Autodesk Inventor part; units mm, degrees
ref_plane "YZ Plane" through (0, 0, 0) normal (1, 0, 0) x (0, 1, 0)
ref_plane "XZ Plane" through (0, 0, 0) normal (0, 1, 0) x (-1, 0, 0)
ref_plane "XY Plane" through (0, 0, 0) normal (0, 0, 1) x (1, 0, 0)
sketch "Sketch1" plane through (0, 0, 0) normal (0, 0, 1) x (1, 0, 0)
  circle A0 centre (-47.5, -10) radius 3
  circle A1 centre (-5, 30) radius 2
  line L0 (-47.5, -10) -> (-2.5, -10)
  line L1 (7.5, 0) -> (-12.5, 0)
  line L2 (-12.5, 0) -> (-12.5, -20)
  line L3 (-12.5, -20) -> (7.5, -20)
  line L4 (7.5, -20) -> (7.5, 0)
  line L5 (7.5, 0) -> (-12.5, -20) construction
  line L6 (-12.5, 0) -> (7.5, -20) construction
  point P0 (0, 0)
  dimension "d0" = 45
  dimension "d1" = 20
  dimension "d2" = 20
extrude "Extrusion1" add sketch "Sketch1" along normal blind 6 contours L4 L3 L2 L1
ref_plane "Work Plane1" through (0, 0, -20) normal (0, 0, -1) x (-1, 0, 0)
sketch "Sketch2" plane through (0, 0, -20) normal (0, 0, -1) x (-1, 0, 0)
  line L0 (-7.5, -20) -> (-7.5, 0)
  line L1 (-7.5, 0) -> (12.5, 0)
  line L2 (12.5, 0) -> (12.5, -20)
  line L3 (12.5, -20) -> (-7.5, -20)
  point P0 (0, 0)
  dimension "d0" = 45
  dimension "d1" = 20
  dimension "d2" = 20
extrude "Extrusion2" add sketch "Sketch2" along normal blind 6
ref_plane "Work Plane2" through (-8, 25, 15) normal (0, 0, 1) x (0, 1, 0)
sketch "Sketch3" plane through (-8, 25, 15) normal (0, 0, 1) x (0, 1, 0)
  circle A0 centre (5, -3) radius 2
  arc A1 (8, -10) -> (10, -8) centre (8, -8) ccw
  line L0 (10, -8) -> (10, -3)
  line L1 (10, -3) -> (10, 5)
  line L2 (0, 5) -> (10, 5)
  line L3 (0, 5) -> (0, -3)
  line L4 (0, -3) -> (0, -8)
  arc A2 (0, -8) -> (2, -10) centre (2, -8) ccw
  line L5 (8, -10) -> (2, -10)
  circle A3 centre (5, -3) radius 2
  line L6 (0, 4) -> (10, 4)
  line L7 (10, 4) -> (10, -10)
  line L8 (10, -10) -> (0, -10)
  line L9 (0, -10) -> (0, 4)
  line L10 (0, 4) -> (10, -10) construction
  line L11 (10, 4) -> (0, -10) construction
  point P0 (-25, -8)
  point P1 (0, -8)
  point P2 (2, -10)
  point P3 (10, -8)
  dimension "d7" = 10
  dimension "d8" = 14
extrude "Extrusion3" add sketch "Sketch3" along normal blind 6
sketch "Sketch4" plane through (-13, 25, 15) normal (0, -1, 0) x (1, 0, 0)
  line L0 (0, 0) -> (15, 0)
  line L1 (15, 0) -> (15, 6)
  line L2 (0, 6) -> (15, 6)
  line L3 (0, 0) -> (0, 6)
  point P0 (13, -15)
sketch "Sketch5" plane through (-12.5, 0, 0) normal (0, 1, 0) x (1, 0, 0)
  line L0 (20, 0) -> (0, 0)
  line L1 (0, 0) -> (0, -6)
  line L2 (20, -6) -> (0, -6)
  line L3 (20, 0) -> (20, -6)
  point P0 (12.5, 0)
loft "Loft1" add section 1 edges at (-2.5, 0, 0) (-12.5, 0, 3) (-2.5, 0, 6) (7.5, 0, 3) section 2 edges at (-5.5, 25, 15) (2, 25, 18) (-5.5, 25, 21) (-13, 25, 18)
ref_plane "Work Plane3" through (0, 0, -10) normal (0, 0, 1) x (1, 0, 0)
mirror "Mirror1" about plane through (0, 0, -10) normal (0, 0, 1) of "Extrusion3", "Loft1"
sketch "Sketch7" plane through (-12.5, -20, 0) normal (0, -1, 0) x (1, 0, 0)
  line L0 (0, 0) -> (20, 0)
  line L1 (20, 0) -> (20, 6)
  line L2 (0, 6) -> (20, 6)
  line L3 (0, 0) -> (0, 6)
  line L4 (20, -20) -> (0, -20)
  line L5 (0, -20) -> (0, -26)
  line L6 (20, -26) -> (0, -26)
  line L7 (20, -20) -> (20, -26)
  line L8 (20, -20) -> (20, -26)
  line L9 (0, 6) -> (20, 6)
  line L10 (20, 6) -> (20, -26)
  line L11 (20, -26) -> (0, -26)
  line L12 (0, -26) -> (0, 6)
  point P0 (12.5, 0)
extrude "Extrusion5" add sketch "Sketch7" along normal blind 5
sketch "Sketch8" plane through (0, 0, 6) normal (0, 0, 1) x (1, 0, 0)
  line L0 (-12.5, -20) -> (7.5, -20)
  line L1 (-2.5, -20) -> (-2.5, -10)
  circle A0 centre (-2.5, -10) radius 3
  point P0 (0, 0)
  dimension "d23" = 10
  dimension "d24" = 6
extrude "Extrusion6" cut sketch "Sketch8" against normal blind 40
fillet "Fillet1" radius 2 2 edges at (2, 35, 18) (2, 35, -38)
fillet "Fillet2" radius 4 2 edges at (-2.5, -25, 6) (-2.5, -25, -26)
sketch "Sketch9" plane through (-12.5, -25, 0) normal (0, -1, 0) x (1, 0, 0)
  line L0 (20, -22) -> (0, -22)
  line L1 (20, -22) -> (20, 2)
  line L2 (0, 2) -> (20, 2)
  line L3 (0, 2) -> (0, -22)
  line L4 (0, 2) -> (0, -22)
  line L5 (0, -22) -> (20, 2)
  line L6 (0, 2) -> (20, 2)
  line L7 (0, 2) -> (20, -22)
  circle A0 centre (10, -10) radius 3
  point P0 (12.5, 0)
  dimension "d29" = 6
extrude "Extrusion7" cut sketch "Sketch9" against normal blind 40 contours A0 L5 L7 | L7 L5 A0 | A0 L7 L5 | L5 L7 A0
properties part number "2020_fixer2"
Could you check a few things on this model? Use its own coordinates, in mm. A direction names the side the tool comes from. Round coordinates to 2 decimals unless told otherwise and drop trailing zeros. Order: outer loops, then holes, each group sorted by start corner. A loop starts at its lowest first (then second) coordinate and runs counter-clockwise, first axis right, second up. Notation, with made-up numbers: M 6.5,26 L 64.5,26 A12 ccw 64.5,38 Z; hole C 60.5,74 d10. An arc over 180 degrees is marked long. One line per question, with ' | ' between items. Start each with the question number.
(1) Please list where these lines run through material, in increasing order: line 1 along Z through (x, y) = (-6.75, -17.5); line 2 along X through (y, z) = (-10, 1.6); line 3 along X through (y, z) = (30, -39.15).
(2) For P1, Ø6.5, axis at x = -5, y = 30, coming from the -Z side; P2, Ø8, axis at x = -2.5, y = -10, coming from the -Z side; P3, Ø5, axis at y = 29, z = -38, coming from the +X side; P4, Ø10, axis at x = 2, y = -14, coming from the +Z side, each with a flat end and sliding along its axis, tell me the tip position at first contact or that it passes through.
(3) Suppose I cut it at A-A on y = 30. List the corners of the cut face in (x, z) for me, then the cut area to 3 significant figures.
(4) Suppose I cut it at B-B on z = -8. List the corners of the cut face in (x, y) for me.
(5) For faces 1 (the face through (-2.36, -23.797, 4.859)), 2 (the face through (2, 29, 18)), 3 (the face through (-5, -8, 0)), which set-ups out of +Z, -Z, +X, -X, +Y, -Y let a thin tool reach every point of the face, with its end or its side?
(6) Thinking about a two-plate mould opening in X: for faces 4 (the face through (-2.891, -7.026, -22.958)), 5 (the face through (0, -13, -26)), 6 (the face through (-13, 30, 18)), 7 (the face through (-4.399, 31.908, 17.958)), which applies, +X half, -X half, draft (parallel to the pull), parting line (faces both ways), or undercut?
(7) Suppose I cut it at C-C on y = -10. List the corners of the cut face in (x, z) for me.
Geometry results:
1) line 1: -26 to -20, 0 to 6 | line 2: -12.5 to -5.5, 0.5 to 7.5 | line 3: -13 to -7, -3 to 2
2) P1: z = -41 | P2: z = -26 | P3: x = 2 | P4: z = 6
3) outline: M -13,-41 L -7,-41 L -7,-35 L -13,-35 Z; M -13,15 L -7,15 L -7,21 L -13,21 Z; M -3,-41 L 2,-41 L 2,-35 L -3,-35 Z; M -3,15 L 2,15 L 2,21 L -3,21 Z | area: 132 mm²
4) outline: M -12.5,-25 L -4.74,-25 L -4.74,-20 L -12.5,-20 Z; M -0.26,-25 L 7.5,-25 L 7.5,-20 L -0.26,-20 Z
5) face 1: +Z, +X, -X, -Y | face 2: +Z, -Z, +X, +Y | face 3: +X, -X, +Y
6) face 4: undercut | face 5: draft | face 6: -X half | face 7: undercut
7) outline: M -12.5,-26 L -5.5,-26 L -5.5,-20 L -12.5,-20 Z; M -12.5,0 L -5.5,0 L -5.5,6 L -12.5,6 Z; M 0.5,-26 L 7.5,-26 L 7.5,-20 L 0.5,-20 Z; M 0.5,0 L 7.5,0 L 7.5,6 L 0.5,6 Z
